The model under review builds one solid part; all positions refer to its coordinate system, in mm. Face numbers are marked on the shaded views. A direction names the side the tool comes from. Give positions to 0.01 mm unless a question says otherwise; leave off trailing zeros. Loops run counter-clockwise (first coordinate to the right, second up) from the corner with the lowest first, then second, coordinate; pieces in that order, holes last. Notation, with made-up numbers: M 46,33.5 L 93,33.5 A10 ccw 93,39.5 Z; hole C -5.75,50 d6. An arc over 180 degrees is marked long. Write item = value, one per line. Start each with the question number.
1. Wall thickness on line 1 along X through (y, z) = (138.5, 13); line 2 along Z through (x, y) = (-29.5, -98.5); line 3 along Y through (x, z) = (-20, 33): over which ranges is each line inside the solid? List them lowest first. Write a range as from..to.
2. We need section A-A on y = -10.5. Give the boundary of the cut face in (x, z), then the cut area to 3 significant figures.
3. We need section C-C on z = 9.5. Give the boundary of the cut face in (x, y).
4. For pin 1 (2.5 mm diameter, centred on y = -61, z = 37.5, fed in from -X); pin 2 (5 mm diameter, centred on x = -27, z = 35, fed in from +Y); pin 3 (1.5 mm diameter, centred on y = 88.5, z = 12.5, fed in from -X), all flat-tipped, find the tip position at first contact; note any pin that passes through.
5. For the marked faces 1, 2, 3 and 4, list the 3-axis set-ups (+Z, -Z, +X, -X, +Y, -Y) from which the entire face can be reached by the end or side of a thin tool; tool diameter is ignored.
6. We need section B-B on x = -4.5. Give the boundary of the cut face in (y, z).
from build123d import *

# Parameters (mm, degrees)
SKETCH1_W           = 20
SKETCH1_H           = 344.8
BOSS_EXTRUDE1_DEPTH = 46
SKETCH2_W           = 6.35
SKETCH2_H           = 290.9
BOSS_EXTRUDE2_DEPTH = 22.9
CUT_EXTRUDE1_DEPTH  = 20
SKETCH2_3_W         = 8.73125
SKETCH2_3_H         = 290.9
BOSS_EXTRUDE3_DEPTH = 15.8


with BuildPart() as part:
    # Sketch1 → Boss-Extrude1 (new body)
    with BuildSketch(Plane.XY):
        Rectangle(SKETCH1_W, SKETCH1_H)
    extrude(amount=BOSS_EXTRUDE1_DEPTH)

    # Sketch2 → Boss-Extrude2 (add)
    with BuildSketch(Plane.ZY.offset(10)):
        with Locations((42.825, 0)):
            Rectangle(SKETCH2_W, SKETCH2_H)
        with Locations((27.74375, 0)):
            Rectangle(SKETCH2_W, SKETCH2_H)
    extrude(amount=BOSS_EXTRUDE2_DEPTH)

    # Sketch3 → Cut-Extrude1 (cut)
    with BuildSketch(Plane.ZY.offset(10)):
        Polygon((46, -172.4), (46, -152.4), (29.491, -152.4), (33.0175, -172.4), align=None)
        Polygon((12.9825, -172.4), (16.509, -152.4), (0, -152.4), (0, -172.4), align=None)
        Polygon((0, 172.4), (0, 152.4), (16.509, 152.4), (12.9825, 172.4), align=None)
        Polygon((29.491, 152.4), (46, 152.4), (46, 172.4), (33.0175, 172.4), align=None)
    extrude(amount=-CUT_EXTRUDE1_DEPTH, mode=Mode.SUBTRACT)

    # Sketch2_3 → Boss-Extrude3 (add)
    with BuildSketch(Plane.ZY.offset(10)):
        with Locations((35.284375, 0)):
            Rectangle(SKETCH2_3_W, SKETCH2_3_H)
    extrude(amount=BOSS_EXTRUDE3_DEPTH)


solid = part.part
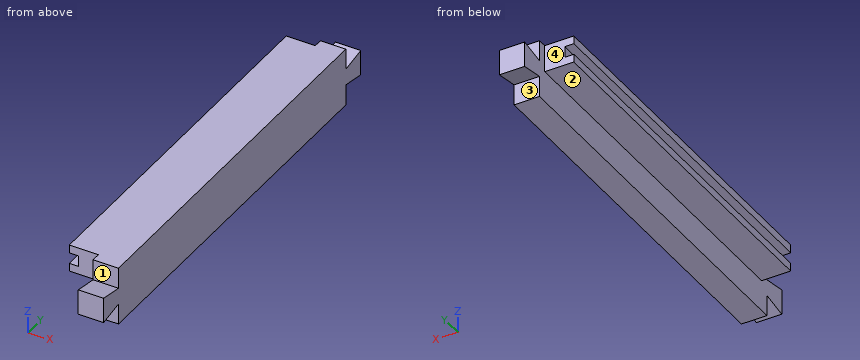
Final values:
q1.line_1 = -10..10
q1.line_2 = 24.57..30.92, 39.65..46
q1.line_3 = -145.45..145.45
q2.outline = M -32.9,24.57 L -10,24.57 L -10,0 L 10,0 L 10,46 L -32.9,46 L -32.9,39.65 L -25.8,39.65 L -25.8,30.92 L -32.9,30.92 Z
q2.area = 1,350 mm²
q3.outline = M -10,-152.4 L 10,-152.4 L 10,152.4 L -10,152.4 Z
q4.pin_1 = -25.8
q4.pin_2 = 145.45
q4.pin_3 = -10
q5.face_1 = +Z, +X, -X
q5.face_2 = -Z, -X, +Y, -Y
q5.face_3 = -Z, +X, -X
q5.face_4 = +Z, -Z, -X, +Y
q6.outline = M -172.4,12.98 L -152.4,16.51 L -152.4,0 L 152.4,0 L 152.4,16.51 L 172.4,12.98 L 172.4,33.02 L 152.4,29.49 L 152.4,46 L -152.4,46 L -152.4,29.49 L -172.4,33.02 Z
